Source: CAD feature listing. Evaluate the final solid. Frame: model axes, mm. A direction names the side the tool comes from. Coordinates: 2 decimals unless noted, no trailing zeros. Loops run counter-clockwise (first coordinate to the right, second up) from the corner with the lowest first, then second, coordinate; pieces in that order, holes last. Notation, with made-up numbers: (58, 88.5) - (103, 88.5) arc R14 cw to (103, 109.5) - close; hole circle Ø7 at (31.25, 62.5). An arc over 180 degrees is marked (long way). Use CSV: the item, a comma, the result in double quotes. Start each with the question number.
```python
from build123d import *

# Parameters (mm, degrees)
BOSS_EXTRUDE1_OUTLINE_R = 67.5
BOSS_EXTRUDE1_DEPTH     = 10
SKETCH4_R               = 5
BOSS_EXTRUDE2_DEPTH     = 90
BOSS_EXTRUDE3_START     = 70
SKETCH4_3_R             = 10
SKETCH4_3_R_2           = 5
BOSS_EXTRUDE3_DEPTH     = 10
BOSS_EXTRUDE4_DEPTH     = 50
SKETCH6_W               = 30
SKETCH6_H               = 61
SKETCH6_W_2             = 22
SKETCH6_H_2             = 41
BOSS_EXTRUDE5_DEPTH     = 20
SKETCH6_7_W             = 22
SKETCH6_7_H             = 41
BOSS_EXTRUDE6_DEPTH     = 20
SKETCH6_3_W             = 22
SKETCH6_3_H             = 41
CUT_EXTRUDE1_DEPTH      = 166.583644089
CIRPATTERN1_COUNT       = 3


# Read off the part's stored shape, not the designer's step: Boss-Extrude1
with BuildPart() as part:
    # Boss-Extrude1 outline → Boss-Extrude1 (new body)
    with BuildSketch(Plane(origin=(0, 0, 0), x_dir=(1, 0, 0), z_dir=(0, 1, 0))):
        Circle(BOSS_EXTRUDE1_OUTLINE_R)
    extrude(amount=BOSS_EXTRUDE1_DEPTH)

    # Sketch4 → Boss-Extrude2 (add)
    with BuildSketch(Plane(origin=(0, 10, 0), x_dir=(1, 0, 0), z_dir=(0, 1, 0))):
        with Locations(Location((47.631397208, 27.5, 0), (0, 0, 90))):
            Circle(SKETCH4_R)
    boss_extrude2 = extrude(amount=BOSS_EXTRUDE2_DEPTH)

    # Sketch4<3> → Boss-Extrude3 (add)
    with BuildSketch(Plane(origin=(0, 10, 0), x_dir=(1, 0, 0), z_dir=(0, 1, 0)).offset(BOSS_EXTRUDE3_START)):
        with Locations(Location((47.631397208, 27.5, 0), (0, 0, 270))):
            Circle(SKETCH4_3_R)
        with Locations(Location((47.631397208, 27.5, 0), (0, 0, 90))):
            Circle(SKETCH4_3_R_2, mode=Mode.SUBTRACT)
    boss_extrude3 = extrude(amount=BOSS_EXTRUDE3_DEPTH)

    # Sketch5 → Boss-Extrude4 (add)
    with BuildSketch(Plane(origin=(0, 10, 0), x_dir=(1, 0, 0), z_dir=(0, 1, 0))):
        Polygon((12.520884891, 39.12285698), (16.056418797, 42.658390886), (30.19855442, 28.516255262), (26.663020514, 24.980721356), align=None)
    boss_extrude4 = extrude(amount=BOSS_EXTRUDE4_DEPTH)

    # Sketch6 → Boss-Extrude5 (add)
    with BuildSketch(Plane(origin=(25.821870935, 0, -25.821870935), x_dir=(0.7071067811865516, 0, 0.7071067811865435), z_dir=(-0.7071067811865435, 0, 0.7071067811865516))):
        with Locations((-8.810434857, 40.5)):
            Rectangle(SKETCH6_W, SKETCH6_H)
        with Locations((-8.810434857, 40.5)):
            Rectangle(SKETCH6_W_2, SKETCH6_H_2, mode=Mode.SUBTRACT)
    boss_extrude5 = extrude(amount=-BOSS_EXTRUDE5_DEPTH)

    # Sketch6<7> → Boss-Extrude6 (add)
    with BuildSketch(Plane(origin=(25.821870935, 0, -25.821870935), x_dir=(0.7071067811865516, 0, 0.7071067811865435), z_dir=(-0.7071067811865435, 0, 0.7071067811865516))):
        with Locations((-8.810434857, 40.5)):
            Rectangle(SKETCH6_7_W, SKETCH6_7_H)
    extrude(amount=-BOSS_EXTRUDE6_DEPTH)

    # Sketch6<3> → Cut-Extrude1 (cut, through all)
    with BuildSketch(Plane(origin=(25.821870935, 0, -25.821870935), x_dir=(0.7071067811865516, 0, 0.7071067811865435), z_dir=(-0.7071067811865435, 0, 0.7071067811865516))):
        with Locations((-8.810434857, 40.5)):
            Rectangle(SKETCH6_3_W, SKETCH6_3_H)
    cut_extrude1 = extrude(amount=-CUT_EXTRUDE1_DEPTH, mode=Mode.SUBTRACT)

    # CirPattern1: Boss-Extrude2, Boss-Extrude3, Boss-Extrude4, Boss-Extrude5, Cut-Extrude1 ×3 about axis
    cirpattern1_axis = Axis((0, 0, 0), (0, 1, 0))
    add([boss_extrude2.rotate(cirpattern1_axis, i * 360 / CIRPATTERN1_COUNT) for i in range(1, CIRPATTERN1_COUNT)])
    add([boss_extrude3.rotate(cirpattern1_axis, i * 360 / CIRPATTERN1_COUNT) for i in range(1, CIRPATTERN1_COUNT)])
    add([boss_extrude4.rotate(cirpattern1_axis, i * 360 / CIRPATTERN1_COUNT) for i in range(1, CIRPATTERN1_COUNT)])
    add([boss_extrude5.rotate(cirpattern1_axis, i * 360 / CIRPATTERN1_COUNT) for i in range(1, CIRPATTERN1_COUNT)])
    add([cut_extrude1.rotate(cirpattern1_axis, i * 360 / CIRPATTERN1_COUNT) for i in range(1, CIRPATTERN1_COUNT)], mode=Mode.SUBTRACT)


solid = part.part
```
(1) Reachability of faces 1 (the flat face through (9.9, 40.2, 45.4)), 2 (the flat face through (31.14, 40.21, 39.67)), 3 (the cylindrical face through (-1.5, 94.93, 50.23)) from +Z, -Z, +X, -X, +Y, -Y: full face, straight path, thin tool, end or side. Return the list, or none.
(2) Draft query along X for faces 4 (the flat face through (-48, 100, -27)), 5 (the flat face through (50, 80, -32.1)), 6 (the cylindrical face through (56.06, 84.93, -22.12)), 7 (the flat face through (24.16, 47.7, -55.77)). Return one class per face: released by +X, released by -X, zero draft, split by the parting line, or undercut.
(3) Section D-D on x = 0. Output: boundary loops of the cut face in (y, z).
(4) Section A-A on z = -2. Output: boundary loops of the cut face in (x, y).
(5) Ray query, line 1 (Y direction, x = 23, z = 35); line 2 (Y direction, x = 7, z = 40.5); line 3 (X direction, y = 36, z = 51). Return the intervals inside material, ascending. Write a range as [from, to].
(6) Pin query (flat end, axial travel): pin 1 Ø6 at (y, z) = (65, 23.5) entering from -X; pin 2 Ø12 at (x, y) = (33, 64.5) entering from -Z; pin 3 Ø21.5 at (x, z) = (-41, -0.5) entering from +Y; pin 4 Ø1.5 at (x, y) = (-2, 75) entering from -Z. Return the tip coordinate at first contact, or that it passes through.
(7) Section C-C on y = 25.5. State how many separate pieces and enclosed holes the cut face has, plus the area to 3 significant figures.
(8) Section B-B on x = 20. Output: boundary loops of the cut face in (y, z), plus the area to 3 significant figures.
Solution:
1,face 1,"none"
1,face 2,"+Z"
1,face 3,"+Y"
2,face 4,"zero draft"
2,face 5,"undercut"
2,face 6,"undercut"
2,face 7,"released by +X"
3,outline,"(0, -67.5) - (10, -67.5) - (10, 50) - (80, 50) - (80, 45) - (90, 45) - (90, 50) - (100, 50) - (100, 60) - (90, 60) - (90, 65) - (80, 65) - (80, 60) - (10, 60) - (10, 67.5) - (0, 67.5) - close"
4,outline,"(-67.47, 0) - (67.47, 0) - (67.47, 10) - (-37.27, 10) - (-37.27, 20) - (-57.98, 20) - (-57.98, 10) - (-67.47, 10) - close; (-57.98, 61) - (-37.27, 61) - (-37.27, 71) - (-57.98, 71) - close"
5,line 1,"y = [0, 20], [61, 71]"
5,line 2,"y = [0, 71]"
5,line 3,"x = [-3, 3], [7.26, 11.4]"
6,pin 1,"passes through"
6,pin 2,"stops at z = -52.93"
6,pin 3,"stops at y = 71"
6,pin 4,"stops at z = 50.16"
7,separate pieces,"9"
7,enclosed holes,"0"
7,area,"716 mm²"
8,outline,"(0, -64.47) - (10, -64.47) - (10, -53.67) - (71, -53.67) - (71, -31.64) - (61, -31.64) - (61, -48.02) - (20, -48.02) - (20, -31.64) - (10, -31.64) - (10, 32.45) - (20, 32.45) - (20, 53.15) - (10, 53.15) - (10, 64.47) - (0, 64.47) - close; (61, 32.45) - (71, 32.45) - (71, 53.15) - (61, 53.15) - close"
8,area,"2,380 mm²"
